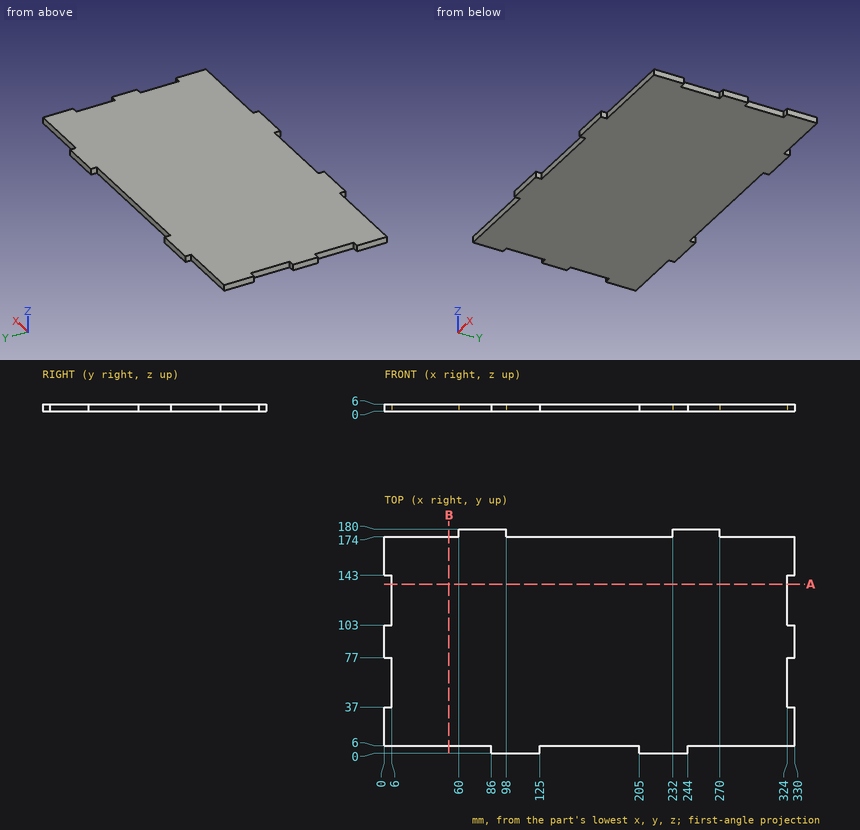
Can you work these out from the drawing? Everything is in mm from the part's minimum corner. Round coordinates to 2 decimals unless told otherwise and drop trailing zeros. Order: outer loops, then holes, each group sorted by start corner. A loop starts at its lowest first (then second) coordinate and runs counter-clockwise, first axis right, second up.
(1) If we section it at B-B (x = 52): Please give me the cut outline in (y, z).
Results are:
outline: (6, 0) - (174, 0) - (174, 6) - (6, 6) - close
(2) If we section it at A-A (y = 136): Please give me the cut outline in (x, z).
Results are:
outline: (6, 0) - (324, 0) - (324, 6) - (6, 6) - close
(3) I'm going to push flat-ended pins straight in: pin 1 (3 mm diameter, centred on y = 176.5, z = 3.5, fed in from +X); pin 2 (1.8 mm diameter, centred on y = 1.5, z = 4, fed in from +X); pin 3 (3 mm diameter, centred on x = 2.5, z = 3, fed in from -Y). Where does each tip first touch, or does it pass through?
Results are:
pin 1: stops at x = 270
pin 2: stops at x = 244
pin 3: stops at y = 6
(4) If I drill on L1, parallel to Y at x = 52, z = 5.7; L2, parallel to X at y = 137, z = 5; L3, parallel to Y at x = 261, z = 0.7, over which ranges is the centre line in solid material (lowest first)?
Results are:
L1: y = 6 to 174
L2: x = 6 to 324
L3: y = 6 to 180
